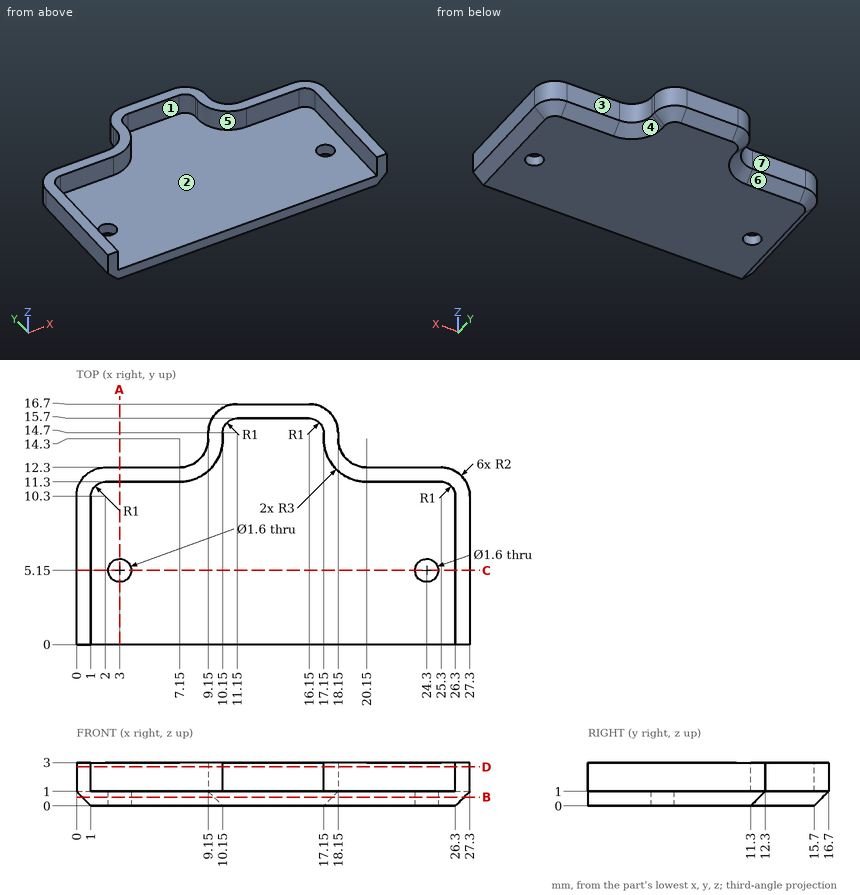
Study the drawing (mm; zero at the part's minimum x, y, z) and answer. A direction names the side the tool comes from. Round coordinates to 2 decimals unless told otherwise and drop trailing zeros. Write each loop counter-clockwise with the first axis right and the second up, starting at its lowest first coordinate (ties: lowest second). Pieces come first, ordered by that corner, then holes.
1) A cutting plane is placed at A-A (x = 3). Give the vertices of the cut face in (y, z), plus the area to 3 significant figures.
2) A cutting plane is placed at D-D (z = 2.7). Give the vertices of the cut face in (x, y).
3) Straight lines are drawn through the part: line 1 (X direction, y = 7.5, z = 1.35); line 2 (Y direction, x = 6, z = 2.1); line 3 (Z direction, x = 11.25, y = 5). For each, find the intervals that lie inside material, in ascending order.
4) A tool of negligible diameter and unlimited length cuts with its end or side. For the marked faces 5, 6 and 7, from which of +Z, -Z, +X, -X, +Y, -Y can it reach the whole face along a straight path? Write none if from no direction.
5) A cutting plane is placed at C-C (y = 5.15). Give the vertices of the cut face in (x, z), plus the area to 3 significant figures.
6) Given pin 1 Ø1 at (x, z) = (14, 2) entering from -Y; pin 2 Ø4 at (x, y) = (3.5, 2) entering from +Z; pin 3 Ø1 at (x, z) = (21.5, 1.5) entering from +Y, each flat-ended and moving along its own axis, determine where each tip first touches the part or whether it passes through.
7) A cutting plane is placed at B-B (z = 0.6). Give the vertices of the cut face in (x, y), plus the area to 3 significant figures.
8) The mould has two halves that part along X. Classify the marked faces 1, 2, 3 and 4: pulls with the +X half, pulls with the -X half, needs draft (parallel to the pull), parting line crosses it, or undercut.
Completed:
1. outline: (0, 0) - (4.35, 0) - (4.35, 1) - (0, 1) - close; (5.95, 0) - (11.3, 0) - (12.3, 1) - (12.3, 3) - (11.3, 3) - (11.3, 1) - (5.95, 1) - close
1. area: 12.2 mm2
2. outline: (0, 0) - (1, 0) - (1, 10.3) arc R1 cw to (2, 11.3) - (7.15, 11.3) arc R3 ccw to (10.15, 14.3) - (10.15, 14.7) arc R1 cw to (11.15, 15.7) - (16.15, 15.7) arc R1 cw to (17.15, 14.7) - (17.15, 14.3) arc R3 ccw to (20.15, 11.3) - (25.3, 11.3) arc R1 cw to (26.3, 10.3) - (26.3, 0) - (27.3, 0) - (27.3, 10.3) arc R2 ccw to (25.3, 12.3) - (20.15, 12.3) arc R2 cw to (18.15, 14.3) - (18.15, 14.7) arc R2 ccw to (16.15, 16.7) - (11.15, 16.7) arc R2 ccw to (9.15, 14.7) - (9.15, 14.3) arc R2 cw to (7.15, 12.3) - (2, 12.3) arc R2 ccw to (0, 10.3) - close
3. line 1: x = 0 to 1, 26.3 to 27.3
3. line 2: y = 11.3 to 12.3
3. line 3: z = 0 to 1
4. face 5: +Z, -Y
4. face 6: -Z, -X, +Y
4. face 7: +Z, -Z, -X, +Y
5. outline: (0, 1) - (1, 0) - (2.2, 0) - (2.2, 1) - (1, 1) - (1, 3) - (0, 3) - close; (3.8, 0) - (23.5, 0) - (23.5, 1) - (3.8, 1) - close; (25.1, 0) - (26.3, 0) - (27.3, 1) - (27.3, 3) - (26.3, 3) - (26.3, 1) - (25.1, 1) - close
5. area: 27.1 mm2
6. pin 1: stops at y = 15.7
6. pin 2: stops at z = 1
6. pin 3: stops at y = 12.3
7. outline: (0.4, 0) - (26.9, 0) - (26.9, 10.3) arc R1.6 ccw to (25.3, 11.9) - (20.15, 11.9) arc R2.4 cw to (17.75, 14.3) - (17.75, 14.7) arc R1.6 ccw to (16.15, 16.3) - (11.15, 16.3) arc R1.6 ccw to (9.55, 14.7) - (9.55, 14.3) arc R2.4 cw to (7.15, 11.9) - (2, 11.9) arc R1.6 ccw to (0.4, 10.3) - close; hole circle Ø1.6 at (3, 5.15); hole circle Ø1.6 at (24.3, 5.15)
7. area: 348 mm2
8. face 1: undercut
8. face 2: undercut
8. face 3: needs draft
8. face 4: pulls with the +X half
